Source: CAD feature listing. Evaluate the final solid. Frame: model axes, mm. A direction names the side the tool comes from. Give positions to 0.01 mm unless a question says otherwise; leave off trailing zeros.
1) Material intervals for line 1 (Y direction, x = 97, z = 7.25); line 2 (Y direction, x = 751, z = -13); line 3 (Z direction, x = 113.5, y = -4), sorted ascending.
2) Section A-A, the plane x = -262. Give the number of separate pieces and of enclosed holes in the cut face, plus the area to 3 significant figures.
3) First-contact query: P1, Ø1.5, axis at x = -326.5, y = -7, coming from the -Z side. Flat tip, straight axial feed; report the tip coordinate or a pass-through.
4) Access query for faces 1 (the face through (771, 7, 0)), 2 (the face through (11, 6, 0)). Directions: +Z, -Z, +X, -X, +Y, -Y. A direction counts if a zero-diameter tool reaches every point of the face in a straight line with its end or side. Return the directions, or none.
```python
from build123d import *

# Parameters (mm, degrees)
SKETCH_1_W             = 23.5
SKETCH_1_H             = 12
EXTRUDE_1_DEPTH        = 771
HOLE_WIZARD_M6_1_D     = 5
HOLE_WIZARD_M6_1_DEPTH = 15
HOLE_WIZARD_M6_1_TIP   = 1.502151548
HOLE_WIZARD_M6_2_D     = 5
HOLE_WIZARD_M6_2_DEPTH = 15
HOLE_WIZARD_M6_2_TIP   = 1.502151548
HOLE_WIZARD_M6_3_D     = 5
HOLE_WIZARD_M6_3_DEPTH = 15
HOLE_WIZARD_M6_3_TIP   = 1.502151548
HOLE_WIZARD_M6_4_D     = 5
HOLE_WIZARD_M6_4_DEPTH = 15
HOLE_WIZARD_M6_4_TIP   = 1.502151548


with BuildPart() as part:
    # 草图1 → 凸台-拉伸1 (new, symmetric)
    with BuildSketch(Plane(origin=(0, 0, 0), x_dir=(0, 0, -1), z_dir=(1, 0, 0))):
        with BuildLine():
            Line((-14, 15), (-11.5, 15))
            Line((-11.5, 15), (-11.5, 13.5))
            Line((-11.5, 13.5), (-11.4, 13.5))
            ThreePointArc((-11.4, 13.5), (-11.117157288, 13.382842712), (-11, 13.1))
            Line((-11, 13.1), (-11, 12))
            Line((-11, 12), (-9.5, 12))
            Line((-9.5, 12), (-9.5, 15))
            Line((-9.5, 15), (-8, 15))
            Line((-8, 15), (-8, 12.5))
            Line((-8, 12.5), (-5, 12.5))
            Line((-5, 12.5), (-5, 15))
            Line((-5, 15), (5, 15))
            Line((5, 15), (5, 12.5))
            Line((5, 12.5), (8, 12.5))
            Line((8, 12.5), (8, 15))
            Line((8, 15), (9.5, 15))
            Line((9.5, 15), (9.5, 12))
            Line((9.5, 12), (11, 12))
            Line((11, 12), (11, 13.1))
            ThreePointArc((11, 13.1), (11.117157288, 13.382842712), (11.4, 13.5))
            Line((11.4, 13.5), (11.5, 13.5))
            Line((11.5, 13.5), (11.5, 15))
            Line((11.5, 15), (14, 15))
            ThreePointArc((14, 15), (14.707106781, 14.707106781), (15, 14))
            Line((15, 14), (15, 8))
            Line((15, 8), (12.5, 8))
            Line((12.5, 8), (12.5, 5))
            Line((12.5, 5), (15, 5))
            Line((15, 5), (15, -5))
            Line((15, -5), (12.5, -5))
            Line((12.5, -5), (12.5, -8))
            Line((12.5, -8), (15, -8))
            Line((15, -8), (15, -14))
            ThreePointArc((15, -14), (14.707106781, -14.707106781), (14, -15))
            Line((14, -15), (11.5, -15))
            Line((11.5, -15), (11.5, -13.5))
            Line((11.5, -13.5), (11.4, -13.5))
            ThreePointArc((11.4, -13.5), (11.117157288, -13.382842712), (11, -13.1))
            Line((11, -13.1), (11, -12))
            Line((11, -12), (9.5, -12))
            Line((9.5, -12), (9.5, -15))
            Line((9.5, -15), (8, -15))
            Line((8, -15), (8, -12.5))
            Line((8, -12.5), (5, -12.5))
            Line((5, -12.5), (5, -15))
            Line((5, -15), (-5, -15))
            Line((-5, -15), (-5, -12.5))
            Line((-5, -12.5), (-8, -12.5))
            Line((-8, -12.5), (-8, -15))
            Line((-8, -15), (-9.5, -15))
            Line((-9.5, -15), (-9.5, -12))
            Line((-9.5, -12), (-11, -12))
            Line((-11, -12), (-11, -13.1))
            ThreePointArc((-11, -13.1), (-11.117157288, -13.382842712), (-11.4, -13.5))
            Line((-11.4, -13.5), (-11.5, -13.5))
            Line((-11.5, -13.5), (-11.5, -15))
            Line((-11.5, -15), (-14, -15))
            ThreePointArc((-14, -15), (-14.707106781, -14.707106781), (-15, -14))
            Line((-15, -14), (-15, 14))
            ThreePointArc((-15, 14), (-14.707106781, 14.707106781), (-14, 15))
        make_face()
        with BuildLine():
            Line((12, -10.5), (12, -8.5))
            ThreePointArc((12, -8.5), (11.853553391, -8.146446609), (11.5, -8))
            Line((11.5, -8), (-11.5, -8))
            ThreePointArc((-11.5, -8), (-11.853553391, -8.146446609), (-12, -8.5))
            Line((-12, -8.5), (-12, -10.5))
            ThreePointArc((-12, -10.5), (-11.853553391, -10.853553391), (-11.5, -11))
            Line((-11.5, -11), (11.5, -11))
            ThreePointArc((11.5, -11), (11.853553391, -10.853553391), (12, -10.5))
        make_face(mode=Mode.SUBTRACT)
        with BuildLine():
            Line((-11.5, 11), (11.5, 11))
            ThreePointArc((11.5, 11), (11.853553391, 10.853553391), (12, 10.5))
            Line((12, 10.5), (12, 8.5))
            ThreePointArc((12, 8.5), (11.853553391, 8.146446609), (11.5, 8))
            Line((11.5, 8), (-11.5, 8))
            ThreePointArc((-11.5, 8), (-11.853553391, 8.146446609), (-12, 8.5))
            Line((-12, 8.5), (-12, 10.5))
            ThreePointArc((-12, 10.5), (-11.853553391, 10.853553391), (-11.5, 11))
        make_face(mode=Mode.SUBTRACT)
        Rectangle(SKETCH_1_W, SKETCH_1_H, mode=Mode.SUBTRACT)
    extrude(amount=EXTRUDE_1_DEPTH, both=True)

    # M6 螺纹孔1
    with Locations(Plane(origin=(0, 15, 0), x_dir=(-1, 0, 0), z_dir=(0, 1, 0))):
        with Locations((-751, 0), (-736, 0), (736, 0), (751, 0)):
            Hole(HOLE_WIZARD_M6_1_D / 2, depth=HOLE_WIZARD_M6_1_DEPTH)
            with Locations((0, 0, -(HOLE_WIZARD_M6_1_DEPTH + HOLE_WIZARD_M6_1_TIP / 2))):  # 118° drill point
                Cone(0, HOLE_WIZARD_M6_1_D / 2, HOLE_WIZARD_M6_1_TIP, mode=Mode.SUBTRACT)

    # M6 螺纹孔2
    with Locations(Plane(origin=(0, 0, -15), x_dir=(-1, 0, 0), z_dir=(0, 0, -1))):
        with Locations((-751, 0), (-736, 0), (736, 0), (751, 0)):
            Hole(HOLE_WIZARD_M6_2_D / 2, depth=HOLE_WIZARD_M6_2_DEPTH)
            with Locations((0, 0, -(HOLE_WIZARD_M6_2_DEPTH + HOLE_WIZARD_M6_2_TIP / 2))):  # 118° drill point
                Cone(0, HOLE_WIZARD_M6_2_D / 2, HOLE_WIZARD_M6_2_TIP, mode=Mode.SUBTRACT)

    # M6 螺纹孔3
    with Locations(Plane.XZ.offset(15)):
        with Locations((751, 0), (736, 0), (-736, 0), (-751, 0)):
            Hole(HOLE_WIZARD_M6_3_D / 2, depth=HOLE_WIZARD_M6_3_DEPTH)
            with Locations((0, 0, -(HOLE_WIZARD_M6_3_DEPTH + HOLE_WIZARD_M6_3_TIP / 2))):  # 118° drill point
                Cone(0, HOLE_WIZARD_M6_3_D / 2, HOLE_WIZARD_M6_3_TIP, mode=Mode.SUBTRACT)

    # M6 螺纹孔4
    with Locations(Plane(origin=(0, 0, -15), x_dir=(-1, 0, 0), z_dir=(0, 0, -1))):
        with Locations((411, 0), (351, 0), (-411, 0), (-351, 0)):
            Hole(HOLE_WIZARD_M6_4_D / 2, depth=HOLE_WIZARD_M6_4_DEPTH)
            with Locations((0, 0, -(HOLE_WIZARD_M6_4_DEPTH + HOLE_WIZARD_M6_4_TIP / 2))):  # 118° drill point
                Cone(0, HOLE_WIZARD_M6_4_D / 2, HOLE_WIZARD_M6_4_TIP, mode=Mode.SUBTRACT)


solid = part.part
```
From the geometry:
1. line 1: y = -12.5 to -11, -8 to -6, 6 to 8, 11 to 12.5
1. line 2: y = -15 to -8, -5 to -2.5, 2.5 to 5, 8 to 15
1. line 3: z = -15 to -11.75, 11.75 to 15
2. separate pieces: 1
2. enclosed holes: 3
2. area: 407 mm2
3. P1: stops at z = -12.5
4. face 1: +Z, -Z, +X, +Y, -Y
4. face 2: +X, -X
